Work out the finished part from the listing and answer in its coordinate system (mm). A direction names the side the tool comes from. Coordinates: 2 decimals unless noted, no trailing zeros. Loops run counter-clockwise (first coordinate to the right, second up) from the corner with the lowest first, then second, coordinate; pieces in that order, holes last. Notation, with made-up numbers: M 57,22.5 L 89,22.5 A23 ccw 89,61.5 Z; hole C -19.75,80.5 d4. An arc over 180 degrees is marked long. Write each question's results on one line, items separated by ' | '.
```python
from build123d import *

# Parameters (mm, degrees)
F1_DEPTH = 12
F2_DEPTH = 2


with BuildPart() as f1:
    # F0 (on Top) → F1 (new body)
    with BuildSketch(Plane.XY):
        with BuildLine():
            ThreePointArc((-38.1583740711, 6.0428159826), (-34.4871523359, 3.9617309979), (-33.0333740711, 0))
            ThreePointArc((-33.0333740711, 0), (-34.4871523359, -3.9617309979), (-38.1583740711, -6.0428159826))
            Line((-38.1583740711, -6.0428159826), (-38.1583740711, -6.125))
            Line((-38.1583740711, -6.125), (-38.1583740711, -8.2192253321))
            Line((-38.1583740711, -8.2192253321), (-40.1583740711, -8.2192253321))
            Line((-40.1583740711, -8.2192253321), (-40.1583740711, -6.2192253321))
            Line((-40.1583740711, -6.2192253321), (-40.1583740711, -6.0428159826))
            ThreePointArc((-40.1583740711, -6.0428159826), (-45.2833740711, 0), (-40.1583740711, 6.0428159826))
            Line((-40.1583740711, 6.0428159826), (-40.1583740711, 6.125))
            Line((-40.1583740711, 6.125), (-40.1583740711, 9.9498743711))
            ThreePointArc((-40.1583740711, 9.9498743711), (-45.8665780036, -7.4161984871), (-29.1583740711, 0))
            ThreePointArc((-29.1583740711, 0), (-31.742175584, 6.7082039325), (-38.1583740711, 9.9498743711))
            Line((-38.1583740711, 9.9498743711), (-38.1583740711, 6.125))
            Line((-38.1583740711, 6.125), (-38.1583740711, 6.0428159826))
        make_face()
    extrude(amount=F1_DEPTH)

    # F0 (on Top) → F2 (join)
    with BuildSketch(Plane.XY):
        with BuildLine():
            Line((-38.1583740711, 12.4599357944), (-38.1583740711, 9.9498743711))
            ThreePointArc((-38.1583740711, 9.9498743711), (-31.742175584, 6.7082039325), (-29.1583740711, 0))
            ThreePointArc((-29.1583740711, 0), (-45.8665780036, -7.4161984871), (-40.1583740711, 9.9498743711))
            Line((-40.1583740711, 9.9498743711), (-40.1583740711, 12.4599357944))
            ThreePointArc((-40.1583740711, 12.4599357944), (-47.63628655, -9.1855865354), (-26.6583740711, 0))
            ThreePointArc((-26.6583740711, 0), (-29.9727875357, 8.4779124789), (-38.1583740711, 12.4599357944))
        make_face()
    extrude(amount=F2_DEPTH)


solid = f1.part
```
1) Find section A-A, the plane x = -44. Give the vertices of the cut face in (y, z).
Check result:
outline: M -11.52,0 L -3.75,0 L -3.75,12 L -8.75,12 L -8.75,2 L -11.52,2 Z; M 3.75,0 L 11.52,0 L 11.52,2 L 8.75,2 L 8.75,12 L 3.75,12 Z
2) For a pull along X with two mould halves and no side action, classify faces 5 (the face through (-38.158, -7, 6)), 6 (the face through (-35, 5, 12)) as released by +X, released by -X, zero draft, split by the parting line, or undercut.
Check result:
face 5: undercut | face 6: zero draft
3) Given pin 1 Ø1.7 at (y, z) = (-7, 4) entering from -X; pin 2 Ø2.5 at (y, z) = (-7, 8.5) entering from +X; pin 3 Ø4 at (y, z) = (1.5, 6) entering from -X; pin 4 Ø6 at (x, y) = (-45, -5.5) entering from -Z, each flat-ended and moving along its own axis, determine where each tip first touches the part or whether it passes through.
Check result:
pin 1: x = -47.04 | pin 2: x = -30.98 | pin 3: x = -49.16 | pin 4: z = 0
4) Find section D-D, the plane x = -39.25. Give the vertices of the cut face in (y, z), and give its area (3 significant figures).
Check result:
outline: M -12.5,0 L -8.22,0 L -8.22,12 L -10,12 L -10,2 L -12.5,2 Z | area: 26.4 mm^2
5) Find section B-B, the plane z = 6. Give the vertices of the cut face in (x, y) (3 decimals), and give its area (3 significant figures).
Check result:
outline: M -40.158,-8.219 L -40.158,-6.043 A6.125 cw -40.158,6.043 L -40.158,9.95 A10 ccw long -38.158,9.95 L -38.158,6.043 A6.125 cw -38.158,-6.043 L -38.158,-8.219 Z | area: 184 mm^2
6) Which of the six approach directions +Z, -Z, +X, -X, +Y, -Y give full straight-line access (tool end or side, diameter ignored) to faces 1 (the face through (-45.282, -0.121, 5.916)), 2 (the face through (-40.158, -7, 6)), 3 (the face through (-37, 6, 0)), 4 (the face through (-48, 6, 2))?
Check result:
face 1: +Z, -Z | face 2: +Z, -Z, +Y | face 3: -Z, +X, -X, +Y, -Y | face 4: +Z
7) Find section C-C, the plane y = 8.5. Give the vertices of the cut face in (x, z).
Check result:
outline: M -48.32,0 L -40.16,0 L -40.16,12 L -44.43,12 L -44.43,2 L -48.32,2 Z; M -38.16,0 L -29.99,0 L -29.99,2 L -33.89,2 L -33.89,12 L -38.16,12 Z
8) Straight lines are drawn through the part: probe 1 along X at (y, z) = (-0.25, 11.25); probe 2 along X at (y, z) = (7.5, 1.75); probe 3 along Z at (x, y) = (-29.75, -6.75). For each, find the intervals that lie inside material, in ascending order. Write a range as [from, to].
Check result:
probe 1: [-49.16, -45.28], [-33.04, -29.16] | probe 2: [-49.16, -40.16], [-38.16, -29.16] | probe 3: [0, 2]
